from build123d import *

# Parameters (mm, degrees)
CROSSRECESS_DEPTH = 0.75
DRAFT9_ANGLE      = 30
FILLET5_R         = 0.3
SKETCH10_W        = 0.45
SKETCH10_H        = 1.25


with BuildPart() as part:
    # Sketch1 → Base (revolve)
    with BuildSketch(Plane.XY):
        Polygon((16, 1.25), (2.4, 1.25), (1.5, 1.25), (0.55, 2.2), (0, 2.2), (0, 0), (16, 0), align=None)
    revolve(axis=Axis((4.515812911, 0, 0), (-1, 0, 0)))

    # Sketch6 → CrossRecess (cut)
    with BuildSketch(Plane(origin=(0, 0, 0), x_dir=(0, 0, -1), z_dir=(1, 0, 0))):
        Polygon((0.29, 0.29), (0.29, 1.45), (-0.29, 1.45), (-0.29, 0.29), (-1.45, 0.29), (-1.45, -0.29), (-0.29, -0.29), (-0.29, -1.45), (0.29, -1.45), (0.29, -0.29), (1.45, -0.29), (1.45, 0.29), align=None)
    extrude(amount=CROSSRECESS_DEPTH, mode=Mode.SUBTRACT)

    # Draft9
    draft9_faces = [part.faces().sort_by_distance(p)[0] for p in [
        (0.375, -1.45, 0),
        (0.375, 0, 1.45),
        (0.375, 0, -1.45),
        (0.375, 1.45, 0),
    ]]
    draft(draft9_faces, Plane(origin=(0, 2.2, 0), x_dir=(0, 0, -1), z_dir=(-1, 0, 0)), DRAFT9_ANGLE)

    # Fillet5
    fillet5_edges = [part.edges().sort_by_distance(p)[0] for p in [
        (0.375, 0.29, 0.29),
        (0.375, -0.29, 0.29),
        (0.375, -0.29, -0.29),
        (0.375, 0.29, -0.29),
    ]]
    fillet(fillet5_edges, radius=FILLET5_R)

    # Sketch10 → Revolve2 (revolve)
    with BuildSketch(Plane.XY):
        with Locations((1.725, 0.625)):
            Rectangle(SKETCH10_W, SKETCH10_H)
    revolve(axis=Axis((62.228915663, 0, 0), (-1, 0, 0)))


solid = part.part
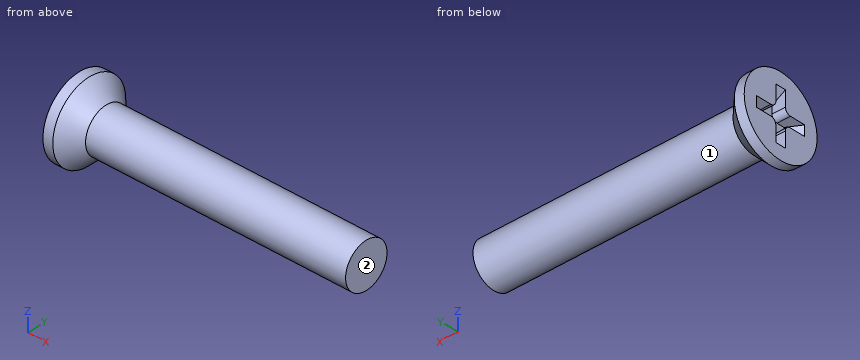
Read the model definition and answer for the solid it produces. Units are mm, in the model's axes. Face numbers are marked on the shaded views. A direction names the side the tool comes from. Round coordinates to 2 decimals unless told otherwise and drop trailing zeros. Order: outer loops, then holes, each group sorted by start corner. A loop starts at its lowest first (then second) coordinate and runs counter-clockwise, first axis right, second up.
1) Straight lines are drawn through the part: L1, parallel to Z at x = 3, y = 0.05; L2, parallel to X at y = 0.5, z = -0.25; L3, parallel to Z at x = 6.5, y = 1.1. For each, find the intervals that lie inside material, in ascending order.
2) The part is cut by section C-C on x = 7.5. Write down the section's boundary in (y, z).
3) The part is cut by section A-A on z = 0. Write down the section's boundary in (x, y), plus the area to 3 significant figures.
4) Flat-ended cylindrical pins translate along their axes: pin 1 (0.8 mm diameter, centred on x = 0.5, y = 1, fed in from +Z); pin 2 (0.8 mm diameter, centred on x = 0.5, z = -1, fed in from -Y); pin 3 (1.5 mm diameter, centred on x = 4, z = 1, fed in from +Y); pin 4 (0.6 mm diameter, centred on y = -0.5, z = -0.5, fed in from -X). Find the tip coordinate at first contact, or state that the pin passes through.
5) For the marked faces 1 and 2, determine the directions among +Z, -Z, +X, -X, +Y, -Y from which every point of the face is accessible in a straight line to the end or side of a thin tool.
Resolved:
1. L1: z = -1.25 to 1.25
1. L2: x = 0.75 to 16
1. L3: z = -0.59 to 0.59
2. outline: circle Ø2.5 at (0, 0)
3. outline: (0, -2.2) - (0.55, -2.2) - (1.5, -1.25) - (16, -1.25) - (16, 1.25) - (1.5, 1.25) - (0.55, 2.2) - (0, 2.2) - (0, 1.45) - (0.75, 1.02) - (0.75, -1.02) - (0, -1.45) - close
3. area: 40.1 mm2
4. pin 1: stops at z = 2.12
4. pin 2: stops at y = -2.12
4. pin 3: stops at y = 1.22
4. pin 4: stops at x = 0
5. face 1: +X
5. face 2: +Z, -Z, +X, +Y, -Y
